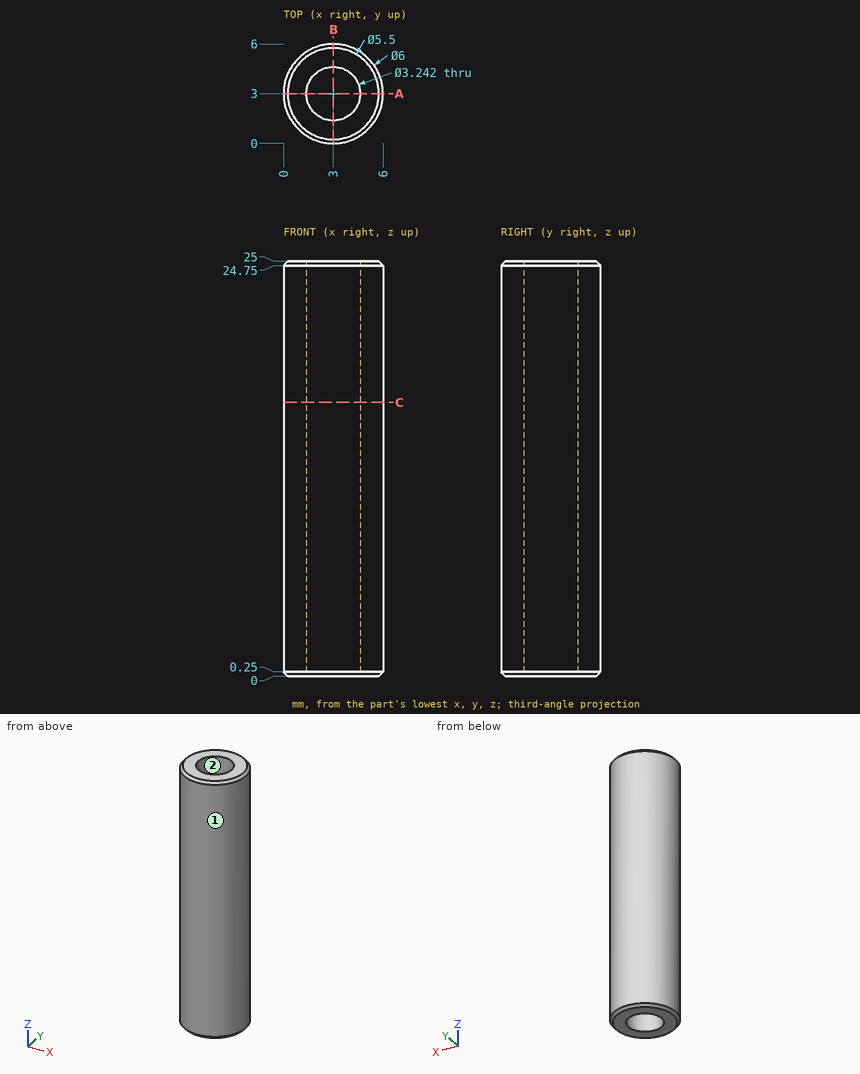
Geometry: see drawing. Coordinates: mm, zero at the bounding-box minimum. Give positions to 0.01 mm unless a question says otherwise; leave off trailing zeros. Write each loop counter-clockwise with the first axis right and the second up, starting at its lowest first coordinate (ties: lowest second). Pieces come first, ordered by that corner, then holes. Notation, with made-up numbers: M -11,-36.75 L 48,-36.75 A32 cw 48,-4.75 Z; hole C -21,-27.5 d5. An arc over 180 degrees is marked long. Return JSON: item names as keys, results as strings. Group by question number.
1) First-contact query: pin 1 Ø1.5 at (y, z) = (4.5, 21) entering from +X; pin 2 Ø1.5 at (y, z) = (2.5, 13) entering from +X; pin 3 Ø1.9 at (x, y) = (3, 3) entering from -Z; pin 4 Ø2 at (x, z) = (4.5, 5) entering from +Y. Flat tips, straight axial feed; report the tip coordinate or a pass-through.
2) Draft query along X for the marked faces 1 and 2. Return one class per face: released by +X, released by -X, zero draft, split by the parting line, or undercut.
3) Cut plane C-C, the plane z = 16.5. Output: boundary loops of the cut face in (x, y), then the cut area to 3 significant figures.
4) Ray query, L1, parallel to Y at x = 3, z = 5.5; L2, parallel to X at y = 2.25, z = 19; L3, parallel to X at y = 1.7, z = 11.5. Return the intervals inside material, ascending.
5) Cut plane A-A, the plane y = 3. Output: boundary loops of the cut face in (x, z).
Data:
{
 "1": {"pin 1": "stops at x = 5.9", "pin 2": "stops at x = 6", "pin 3": "passes through", "pin 4": "stops at y = 5.96"},
 "2": {"face 1": "split by the parting line", "face 2": "undercut"},
 "3": {"outline": "C 3,3 d6; hole C 3,3 d3.24", "area": "20.0 mm²"},
 "4": {"L1": "y = 0 to 1.38, 4.62 to 6", "L2": "x = 0.1 to 1.56, 4.44 to 5.9", "L3": "x = 0.3 to 2.03, 3.97 to 5.7"},
 "5": {"outline": "M 0,0.25 L 0.25,0 L 1.38,0 L 1.38,25 L 0.25,25 L 0,24.75 Z; M 4.62,0 L 5.75,0 L 6,0.25 L 6,24.75 L 5.75,25 L 4.62,25 Z"}
}
